```python
from build123d import *

# Parameters (mm, degrees)
CROQUIS1_R              = 9
SALIENTE_EXTRUIR1_DEPTH = 15


with BuildPart() as part:
    # Croquis1 → Saliente-Extruir1 (new body)
    with BuildSketch(Plane.XY):
        Polygon((-292.5, 0), (292.5, 0), (292.5, 30), (177.5, 30), (177.5, 53), (127.5, 53), (127.5, 30), (62.5, 30), (62.5, 53), (12.5, 53), (12.5, 30), (-52.5, 30), (-52.5, 53), (-102.5, 53), (-102.5, 30), (-292.5, 30), align=None)
        with Locations((37.5, 30.5)):
            Circle(CROQUIS1_R, mode=Mode.SUBTRACT)
        with Locations((-77.5, 30.5)):
            Circle(CROQUIS1_R, mode=Mode.SUBTRACT)
        with Locations((152.5, 30.5)):
            Circle(CROQUIS1_R, mode=Mode.SUBTRACT)
    extrude(amount=SALIENTE_EXTRUIR1_DEPTH)


solid = part.part
```
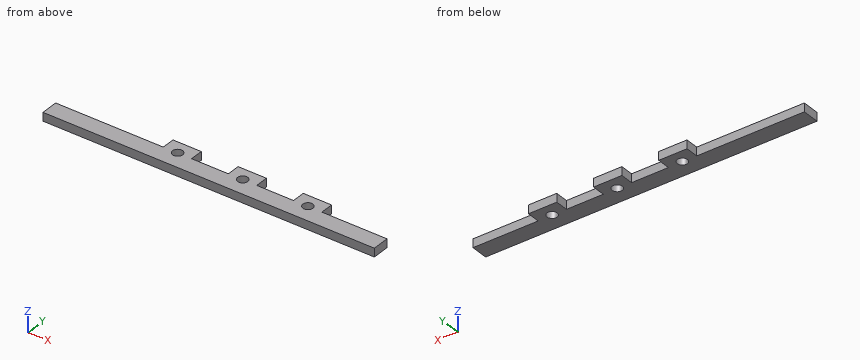
The model under review builds one solid part; all positions refer to its coordinate system, in mm. Round coordinates to 2 decimals unless told otherwise and drop trailing zeros. Write each loop counter-clockwise with the first axis right and the second up, starting at its lowest first coordinate (ties: lowest second). Pieces come first, ordered by that corner, then holes. Notation, with made-up numbers: M 33,70.5 L 41,70.5 A27 cw 41,100.5 Z; hole C 68.25,88 d2. An arc over 180 degrees is marked long. Use CSV: the item, a comma, the result in double quotes. Start each with the question number.
(1) We need section D-D, the plane x = -182. State the section outline as (y, z) points, then the cut area to 3 significant figures.
(2) We need section A-A, the plane y = 44.5. State the section outline as (x, z) points, then the cut area to 3 significant figures.
(3) We need section B-B, the plane x = 37.5. State the section outline as (y, z) points.
(4) Clearance check with flat-ended pins moving along their axes: P1, Ø4, axis at y = 36, z = 3, coming from the +X side; P2, Ø7.5, axis at x = -218, z = 4, coming from the +Y side; P3, Ø4.5, axis at y = 41.5, z = 5.5, coming from the -X side. State where each tip first meets the part, or that it passes through.
(5) For line 1 along Y through (x, z) = (152.5, 9); line 2 along X through (y, z) = (38, 1.25); line 3 along X through (y, z) = (25, 6.25), list the stretches that pass through material, from the lowest coordinate up.
(6) We need section C-C, the plane z = 10.25. State the section outline as (x, y) points.
Findings:
1,outline,"M 0,0 L 30,0 L 30,15 L 0,15 Z"
1,area,"450 mm^2"
2,outline,"M -102.5,0 L -52.5,0 L -52.5,15 L -102.5,15 Z; M 12.5,0 L 62.5,0 L 62.5,15 L 12.5,15 Z; M 127.5,0 L 177.5,0 L 177.5,15 L 127.5,15 Z"
2,area,"2,250 mm^2"
3,outline,"M 0,0 L 21.5,0 L 21.5,15 L 0,15 Z; M 39.5,0 L 53,0 L 53,15 L 39.5,15 Z"
4,P1,"x = 177.5"
4,P2,"y = 30"
4,P3,"x = -102.5"
5,line 1,"0 to 21.5, 39.5 to 53"
5,line 2,"-102.5 to -82.47, -72.53 to -52.5, 12.5 to 32.53, 42.47 to 62.5, 127.5 to 147.53, 157.47 to 177.5"
5,line 3,"-292.5 to -84.62, -70.38 to 30.38, 44.62 to 145.38, 159.62 to 292.5"
6,outline,"M -292.5,0 L 292.5,0 L 292.5,30 L 177.5,30 L 177.5,53 L 127.5,53 L 127.5,30 L 62.5,30 L 62.5,53 L 12.5,53 L 12.5,30 L -52.5,30 L -52.5,53 L -102.5,53 L -102.5,30 L -292.5,30 Z; hole C -77.5,30.5 d18; hole C 37.5,30.5 d18; hole C 152.5,30.5 d18"
